Source: CAD feature listing. Evaluate the final solid. Frame: model axes, mm. Face numbers are marked on the shaded views. Give positions to 0.01 mm unless a question says otherwise; leave off trailing zeros. Order: outer loops, then holes, each group sorted by start corner. A loop starts at its lowest first (then second) coordinate and runs counter-clockwise, first axis right, second up. Notation, with made-up numbers: (-20, 8) - (-11, 8) arc R21 cw to (-11, 41) - close; hole circle Ø8 at (26, 68). An arc over 180 degrees is marked (long way). Answer as CSV lines item,"result".
```python
from build123d import *

# Parameters (mm, degrees)
F0_W      = 666.75
F0_H      = 635
F1_DEPTH  = 165.1
F4_W      = 333.375
F4_H      = 69.85
F5_DEPTH  = 666.751
F6_W      = 635
F6_H      = 63.5
F6_H_2    = 107.95
F6_H_3    = 69.85
F7_DEPTH  = 330.2
F9_DEPTH  = 38.1
F11_DEPTH = 25.4
F13_DEPTH = 25.4
F14_W     = 635
F14_H     = 577.849984169
F15_DEPTH = 31.75
F17_DEPTH = 25.4
F19_D     = 3.175
F19_DEPTH = 38.1
F19_TIP   = 0.9538662327


with BuildPart() as f1:
    # F0 (on Top) → F1 (new body, symmetric)
    with BuildSketch(Plane.XY):
        Rectangle(F0_W, F0_H)
    extrude(amount=F1_DEPTH, both=True)

    # F4 (on face) → F5 (cut, through all)
    with BuildSketch(Plane.YZ.offset(333.375)):
        Polygon((0, 127), (-142.2031428718, 127), (-166.6875, 73.3921443929), (-166.6875, 63.5), (166.6875, 63.5), (166.6875, 73.3921443929), (142.2031428718, 127), align=None)
        Polygon((-166.6875, 63.5), (-166.6875, 73.3921443929), (-171.2055467179, 63.5), align=None)
        Polygon((171.2055467179, 63.5), (166.6875, 73.3921443929), (166.6875, 63.5), align=None)
        Polygon((174.1057871025, 57.15), (166.6875, 57.15), (166.6875, -12.7), (206.0084313333, -12.7), align=None)
        with Locations((0, 22.225)):
            Rectangle(F4_W, F4_H)
        Polygon((-166.6875, -12.7), (-166.6875, 57.15), (-174.1057871025, 57.15), (-206.0084313333, -12.7), align=None)
        Polygon((-208.9086717179, -19.05), (-258.2127582564, -127), (-166.6875, -127), (-166.6875, -19.05), align=None)
        Polygon((-166.6875, -19.05), (-166.6875, -127), (0, -127), (166.6875, -127), (166.6875, -19.05), align=None)
        Polygon((166.6875, -19.05), (166.6875, -127), (258.2127582564, -127), (208.9086717179, -19.05), align=None)
        Polygon((317.5, 165.1), (166.6875, 165.1), (184.0889423077, 127), (213.0913461538, 63.5), (317.5, -165.1), align=None)
        Polygon((-184.0889423077, 127), (-166.6875, 165.1), (-317.5, 165.1), (-317.5, -165.1), (-213.0913461538, 63.5), align=None)
    extrude(amount=-F5_DEPTH, mode=Mode.SUBTRACT)

    # F6 (on Front) → F7 (cut, symmetric)
    with BuildSketch(Plane.XZ):
        with Locations((0, 95.25)):
            Rectangle(F6_W, F6_H)
        with Locations((0, -73.025)):
            Rectangle(F6_W, F6_H_2)
        with Locations((0, 22.225)):
            Rectangle(F6_W, F6_H_3)
    extrude(amount=F7_DEPTH, both=True, mode=Mode.SUBTRACT)

    # F3 (on face) + F8 (on face) → F9 (cut)
    with BuildSketch(Plane.XY.offset(165.1)):
        with BuildLine():
            ThreePointArc((-166.6875, 153.9875), (-320.675, 0), (-166.6875, -153.9875))
            Line((-166.6875, -153.9875), (-166.6875, 153.9875))
        make_face()
        with BuildLine():
            Line((-166.6875, 153.9875), (-166.6875, -153.9875))
            ThreePointArc((-166.6875, -153.9875), (-57.801894532, -108.885605468), (-12.7, 0))
            ThreePointArc((-12.7, 0), (-57.801894532, 108.885605468), (-166.6875, 153.9875))
        make_face()
        with BuildLine():
            ThreePointArc((166.6875, 153.9875), (12.7, 0), (166.6875, -153.9875))
            Line((166.6875, -153.9875), (166.6875, 153.9875))
        make_face()
    with BuildSketch(Plane.XY.offset(165.1)):
        with BuildLine():
            Line((166.6875, 153.9875), (166.6875, -153.9875))
            ThreePointArc((166.6875, -153.9875), (275.573105468, -108.885605468), (320.675, 0))
            ThreePointArc((320.675, 0), (275.573105468, 108.885605468), (166.6875, 153.9875))
        make_face()
    extrude(amount=-F9_DEPTH, mode=Mode.SUBTRACT)

    # F10 (on face) → F11 (cut)
    with BuildSketch(Plane.XY.offset(63.5)):
        with BuildLine():
            ThreePointArc((-166.6875, 127), (-293.6875, 0), (-166.6875, -127))
            Line((-166.6875, -127), (-166.6875, 127))
        make_face()
        with BuildLine():
            Line((-166.6875, 127), (-166.6875, -127))
            ThreePointArc((-166.6875, -127), (-76.8849387893, -89.8025612107), (-39.6875, 0))
            ThreePointArc((-39.6875, 0), (-76.8849387893, 89.8025612107), (-166.6875, 127))
        make_face()
        with BuildLine():
            ThreePointArc((166.6875, 127), (39.6875, 0), (166.6875, -127))
            Line((166.6875, -127), (166.6875, 127))
        make_face()
        with BuildLine():
            Line((166.6875, 127), (166.6875, -127))
            ThreePointArc((166.6875, -127), (256.4900612107, -89.8025612107), (293.6875, 0))
            ThreePointArc((293.6875, 0), (256.4900612107, 89.8025612107), (166.6875, 127))
        make_face()
    extrude(amount=-F11_DEPTH, mode=Mode.SUBTRACT)

    # F12 (on face) → F13 (cut)
    with BuildSketch(Plane.XY.offset(-12.7)):
        with BuildLine():
            ThreePointArc((-166.6875, 57.15), (-223.8375, 0), (-166.6875, -57.15))
            Line((-166.6875, -57.15), (-166.6875, 57.15))
        make_face()
        with BuildLine():
            Line((-166.6875, 57.15), (-166.6875, -57.15))
            ThreePointArc((-166.6875, -57.15), (-126.2763474552, -40.4111525448), (-109.5375, 0))
            ThreePointArc((-109.5375, 0), (-126.2763474552, 40.4111525448), (-166.6875, 57.15))
        make_face()
        with BuildLine():
            ThreePointArc((166.6875, 57.15), (109.5375, 0), (166.6875, -57.15))
            Line((166.6875, -57.15), (166.6875, 57.15))
        make_face()
        with BuildLine():
            Line((166.6875, 57.15), (166.6875, -57.15))
            ThreePointArc((166.6875, -57.15), (207.0986525448, -40.4111525448), (223.8375, 0))
            ThreePointArc((223.8375, 0), (207.0986525448, 40.4111525448), (166.6875, 57.15))
        make_face()
    extrude(amount=-F13_DEPTH, mode=Mode.SUBTRACT)

    # F14 (on face) → F15 (cut)
    with BuildSketch(Plane.XY.offset(-127)):
        Rectangle(F14_W, F14_H)
    extrude(amount=-F15_DEPTH, mode=Mode.SUBTRACT)

    # F16 (on face) → F17 (cut)
    with BuildSketch(Plane.XY.offset(-158.75)):
        with BuildLine():
            ThreePointArc((-166.6875, 25.4), (-192.0875, 0), (-166.6875, -25.4))
            Line((-166.6875, -25.4), (-166.6875, 25.4))
        make_face()
        with BuildLine():
            Line((-166.6875, 25.4), (-166.6875, -25.4))
            ThreePointArc((-166.6875, -25.4), (-148.7269877579, -17.9605122421), (-141.2875, 0))
            ThreePointArc((-141.2875, 0), (-148.7269877579, 17.9605122421), (-166.6875, 25.4))
        make_face()
        with BuildLine():
            Line((166.6875, 25.4), (166.6875, -25.4))
            ThreePointArc((166.6875, -25.4), (184.6480122421, -17.9605122421), (192.0875, 0))
            ThreePointArc((192.0875, 0), (184.6480122421, 17.9605122421), (166.6875, 25.4))
        make_face()
        with BuildLine():
            ThreePointArc((166.6875, 25.4), (141.2875, 0), (166.6875, -25.4))
            Line((166.6875, -25.4), (166.6875, 25.4))
        make_face()
    extrude(amount=-F17_DEPTH, mode=Mode.SUBTRACT)

    # F19
    with Locations(Plane.XY.offset(165.1)):
        with Locations((-6.35, 0), (6.35, 0)):
            Hole(F19_D / 2, depth=F19_DEPTH)
            with Locations((0, 0, -(F19_DEPTH + F19_TIP / 2))):  # 118° drill point
                Cone(0, F19_D / 2, F19_TIP, mode=Mode.SUBTRACT)


solid = f1.part
```
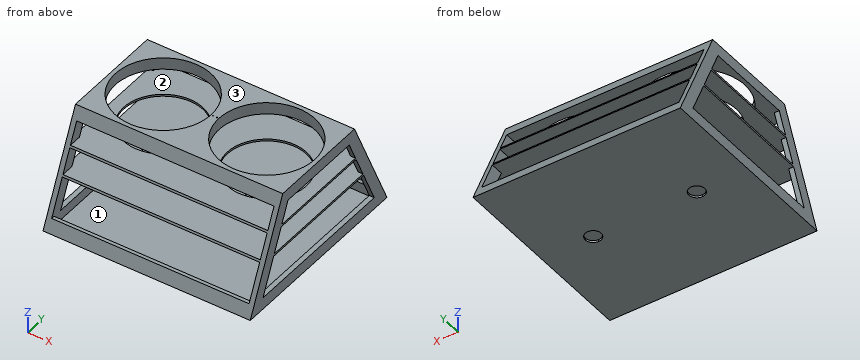
(1) Cut plane C-C (z = 3.5). Return loops of the section in (x, y) (3 decimals), then the cut area to 3 significant figures.
Completed:
outline,"(-333.375, -240.495) - (-317.5, -240.495) - (-317.5, -198.609) - (-333.375, -198.609) - close; (-333.375, 198.609) - (-317.5, 198.609) - (-317.5, 240.495) - (-333.375, 240.495) - close; (317.5, -240.495) - (333.375, -240.495) - (333.375, -198.609) - (317.5, -198.609) - close; (317.5, 198.609) - (333.375, 198.609) - (333.375, 240.495) - (317.5, 240.495) - close"
area,"2,660 mm²"
(2) Mould query, pull axis X, two halves, no side actions, for the marked faces 1, 2 and 3. Classes: released by +X, released by -X, zero draft, split by the parting line, or undercut.
Completed:
face 1,"undercut"
face 2,"undercut"
face 3,"zero draft"
(3) Contact query for flat-ended pins moving along their axis: pin 1 (1.5 mm diameter, centred on x = -27, y = -48, fed in from +Z); pin 2 (3 mm diameter, centred on x = 201, y = -18.5, fed in from +Z); pin 3 (16 mm diameter, centred on x = -8.5, z = -142.5, fed in from +Y). Output: stop coordinate, or through.
Completed:
pin 1,"z = 63.5"
pin 2,"z = -158.75"
pin 3,"y = 310.83"
(4) Cut plane B-B (x = -260.5). Give the number of separate pieces and of enclosed holes in the cut face, then the cut area to 3 significant figures.
Completed:
separate pieces,"6"
enclosed holes,"0"
area,"14,000 mm²"
(5) Cut plane A-A (y = -229). Return loops of the section in (x, z) (3 decimals).
Completed:
outline,"(-333.375, -165.1) - (333.375, -165.1) - (333.375, -127) - (317.5, -127) - (317.5, -158.75) - (-317.5, -158.75) - (-317.5, -127) - (-333.375, -127) - close; (-333.375, -63.039) - (-317.5, -63.039) - (-317.5, -19.05) - (317.5, -19.05) - (317.5, -63.039) - (333.375, -63.039) - (333.375, 28.668) - (317.5, 28.668) - (317.5, -12.7) - (-317.5, -12.7) - (-317.5, 28.668) - (-333.375, 28.668) - close"
(6) Ray query, line 1 (Z direction, x = 234, y = -160); line 2 (Z direction, x = 96, y = -188). Return the intervals inside material, ascending. Write a range as from..to.
Completed:
line 1,"-165.1..-158.75, -19.05..-12.7, 57.15..63.5, 127..165.1"
line 2,"-165.1..-158.75, -19.05..-12.7, 57.15..63.5"
